Part model, mm, in its own coordinate system. A direction names the side the tool comes from. Give positions to 0.01 mm unless a question says otherwise; leave off trailing zeros. Write each loop counter-clockwise with the first axis right and the second up, starting at its lowest first coordinate (ties: lowest second). Pieces come first, ordered by that corner, then holes.
Solid Edge part; units mm, degrees
sketch "Sketch1" plane through (0, 0, 0) normal (0, 0, 1) x (1, 0, 0)
  line L0 (29, 1) -> (29, 59)
  line L1 (29, 59) -> (1, 59)
  line L2 (1, 59) -> (1, 1)
  line L3 (1, 1) -> (29, 1)
  line L4 (30, 0) -> (30, 60)
  line L5 (30, 60) -> (0, 60)
  line L6 (0, 60) -> (0, 0)
  line L7 (0, 0) -> (30, 0)
extrude "Protrusion1" add sketch "Sketch1" along normal blind 400
sketch "Sketch2" plane through (0, 0, 0) normal (0, 0, 1) x (1, 0, 0)
  line L0 (30, 0) -> (30, 60)
  line L1 (30, 60) -> (0, 60)
  line L2 (0, 60) -> (0, 0)
  line L3 (0, 0) -> (30, 0)
  line L4 (29, 1) -> (29, 59)
  line L5 (29, 59) -> (1, 59)
  line L6 (1, 59) -> (1, 1)
  line L7 (1, 1) -> (29, 1)
extrude "ExtrudedProtrusion_6" add sketch "Sketch2" against normal blind 1100
properties material "Galvanized steel"
1) Saw through at A-A, the plane y = 17.5. Write the cut outline in (x, z).
Answers follow:
outline: (0, -1100) - (1, -1100) - (1, 400) - (0, 400) - close; (29, -1100) - (30, -1100) - (30, 400) - (29, 400) - close
2) Saw through at C-C, the plane x = 19.5. Write the cut outline in (y, z).
Answers follow:
outline: (0, -1100) - (1, -1100) - (1, 400) - (0, 400) - close; (59, -1100) - (60, -1100) - (60, 400) - (59, 400) - close
3) 3-axis set-ups, long thin cutter, end or side, ignore diameter. For faces 4 (the face through (0.5, 39, 400)), 5 (the face through (1, 30, -360)): which of +Z, -Z, +X, -X, +Y, -Y reach the whole face in a straight line?
Answers follow:
face 4: +Z, +X, -X, +Y, -Y
face 5: +Z, -Z
4) Pin check, flat tip, straight feed: pin 1 Ø6 at (y, z) = (21.5, -678.5) entering from -X. Stop position of the tip, or through.
Answers follow:
pin 1: stops at x = 0
5) Wall check: L1, parallel to X at y = 9, z = -260.5; L2, parallel to Y at x = 14, z = 23.5. Give the ranges that are in metal, low to high.
Answers follow:
L1: x = 0 to 1, 29 to 30
L2: y = 0 to 1, 59 to 60
6) Two-plate mould, pull along X, no slides. Class faces 1 (the face through (0.5, 39, -1100)), 2 (the face through (15, 59, -360)), 3 (the face through (30, 30, -360)): +X half, -X half, draft (parallel to the pull), parting line (faces both ways), or undercut.
Answers follow:
face 1: draft
face 2: undercut
face 3: +X half
7) Saw through at B-B, the plane z = -687.5. Write the cut outline in (x, y), then the cut area to 3 significant figures.
Answers follow:
outline: (0, 0) - (30, 0) - (30, 60) - (0, 60) - close; hole (1, 1) - (29, 1) - (29, 59) - (1, 59) - close
area: 176 mm2
